The listing builds one solid part. Answer for the finished solid, in the listing's coordinates (mm). Round coordinates to 2 decimals unless told otherwise and drop trailing zeros. Loops run counter-clockwise (first coordinate to the right, second up) from the corner with the lowest first, then second, coordinate; pieces in that order, holes last. Notation, with made-up numbers: (-13.5, 42) - (4.5, 42) arc R10 cw to (4.5, 57) - close; hole circle Ø1 at (-9.5, 28). An arc over 180 degrees is marked (long way). Write item = value, one per line. Start each with the question number.
1) Section D-D, the plane y = 2.5 is taken. Determine the outline of the cut face in (x, z).
2) For a pull along X with two mould halves and no side action, classify faces 1 (the cylindrical face through (2.343, 17.847, 5.916)), 2 (the flat face through (150, 0, 6)), 3 (the flat face through (-2, 30, 6)) as released by +X, released by -X, zero draft, split by the parting line, or undercut.
3) Section C-C, the plane y = -15 is taken. Determine the outline of the cut face in (x, z), and give its area (3 significant figures).
4) Section A-A, the plane x = 100 is taken. Determine the outline of the cut face in (y, z).
5) Section B-B, the plane z = 5.25 is taken. Determine the outline of the cut face in (x, y).
6) Straight lines are drawn through the part: line 1 along Y through (x, z) = (0, 5); line 2 along Y through (x, z) = (100, 9.5); line 3 along X through (y, z) = (3, 8.5). For each, find the intervals that lie inside material, in ascending order.
from build123d import *

# Parameters (mm, degrees)
SKETCH_1_W          = 300
SKETCH_1_H          = 60
SKETCH_1_R          = 12.5
EXTRUDE_1_DEPTH     = 12
CUT_EXTRUDE_1_REACH = 155.441
SKETCH_2_R          = 18


with BuildPart() as part:
    # 草图1 → 凸台-拉伸1 (new body)
    with BuildSketch(Plane.XY):
        Rectangle(SKETCH_1_W, SKETCH_1_H)
        with Locations((100, 0)):
            Circle(SKETCH_1_R, mode=Mode.SUBTRACT)
        with Locations((-100, 0)):
            Circle(SKETCH_1_R, mode=Mode.SUBTRACT)
    extrude(amount=EXTRUDE_1_DEPTH)

    # 草图2 → 切除-拉伸1 (cut, up to next)
    with BuildSketch(Plane(origin=(0, 0, 0), x_dir=(-1, 0, 0), z_dir=(0, 0, -1)), mode=Mode.PRIVATE) as cut_extrude_1_sk1:
        Circle(SKETCH_2_R)
    cut_extrude_1_tool1 = extrude(cut_extrude_1_sk1.sketch, amount=-CUT_EXTRUDE_1_REACH, mode=Mode.PRIVATE) & part.part
    add(cut_extrude_1_tool1.solids().sort_by_distance((0, 0, 0))[0], mode=Mode.SUBTRACT)


solid = part.part
Geometry check:
q1.outline = (-150, 0) - (-112.25, 0) - (-112.25, 12) - (-150, 12) - close; (-87.75, 0) - (-17.83, 0) - (-17.83, 12) - (-87.75, 12) - close; (17.83, 0) - (87.75, 0) - (87.75, 12) - (17.83, 12) - close; (112.25, 0) - (150, 0) - (150, 12) - (112.25, 12) - close
q2.face_1 = undercut
q2.face_2 = released by +X
q2.face_3 = zero draft
q3.outline = (-150, 0) - (-9.95, 0) - (-9.95, 12) - (-150, 12) - close; (9.95, 0) - (150, 0) - (150, 12) - (9.95, 12) - close
q3.area = 3,360 mm2
q4.outline = (-30, 0) - (-12.5, 0) - (-12.5, 12) - (-30, 12) - close; (12.5, 0) - (30, 0) - (30, 12) - (12.5, 12) - close
q5.outline = (-150, -30) - (150, -30) - (150, 30) - (-150, 30) - close; hole circle Ø25 at (-100, 0); hole circle Ø36 at (0, 0); hole circle Ø25 at (100, 0)
q6.line_1 = -30 to -18, 18 to 30
q6.line_2 = -30 to -12.5, 12.5 to 30
q6.line_3 = -150 to -112.13, -87.87 to -17.75, 17.75 to 87.87, 112.13 to 150
